Can you work these out from the drawing? Everything is in mm from the part's minimum corner. Round coordinates to 2 decimals unless told otherwise and drop trailing zeros. Loops run counter-clockwise (first coordinate to the right, second up) from the corner with the lowest first, then second, coordinate; pieces in that order, holes last. Notation, with made-up numbers: (57.25, -3.75) - (100.25, -3.75) arc R10 cw to (100.25, 3.25) - close; hole circle Ø6 at (37.5, 52.25). An arc over 180 degrees is marked (long way). Put each result on its own line as item: value. Start each with the question number.
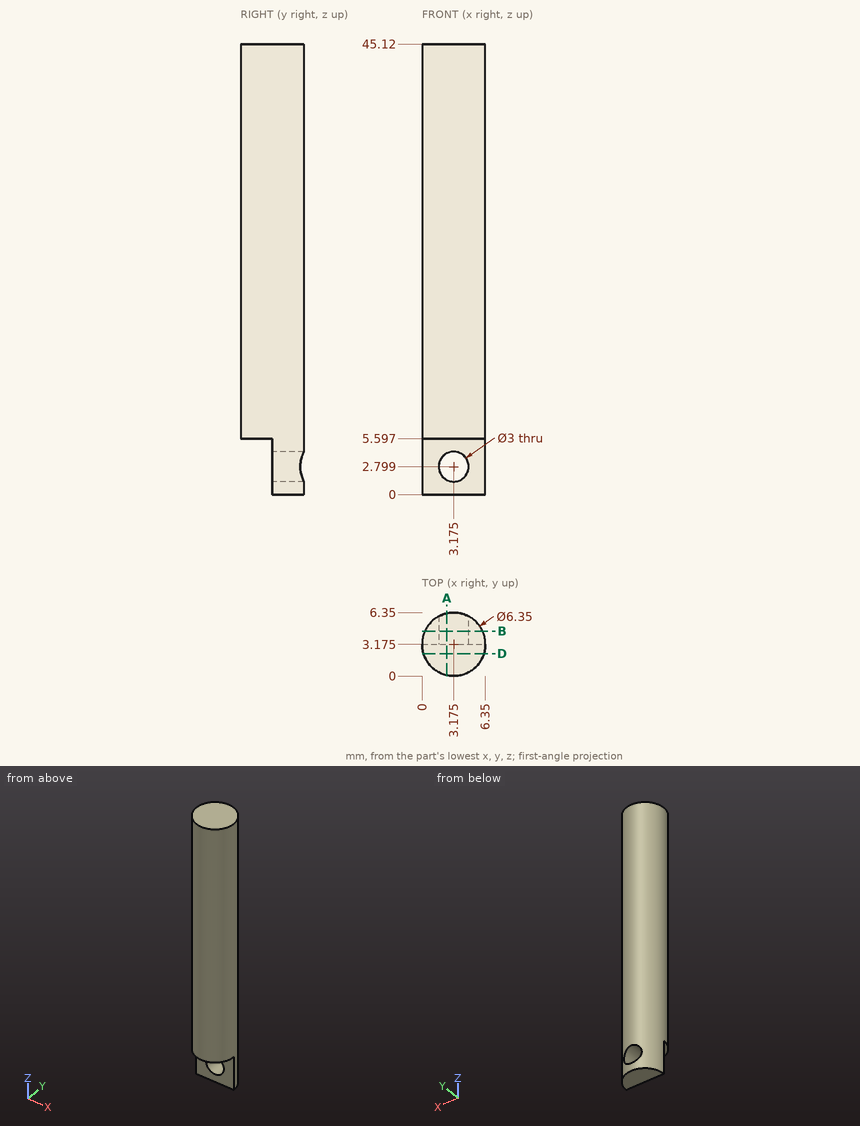
Item 1: Suppose I cut it at A-A, the plane x = 2.5. List the corners of the cut face in (y, z) for me (1 decimal), then the cut area to 3 significant figures.
Item 2: I need wall thicknesses on line 1 (Z direction, x = 1, y = 1.75); line 2 (Z direction, x = 3.75, y = 3.25) (1 decimal); line 3 (Z direction, x = 4.5, y = 3.5) (1 decimal). Which ranges of each line are inside material? Lowest first, please. Write a range as from..to.
Item 3: Suppose I cut it at B-B, the plane y = 4.5. List the corners of the cut face in (x, z) for me (1 decimal), then the cut area to 3 significant figures.
Item 4: Suppose I cut it at D-D, the plane y = 2.25. List the corners of the cut face in (x, z) for me, then the cut area to 3 significant figures.
Item 5: Will these pins go through, and if not, where does the flat tip stop? P1, Ø3.5, axis at x = 3.18, z = 2.8, coming from the -Y side (3 decimals); P2, Ø1, axis at x = 2.5, y = 1, coming from the -Z side; P3, Ø3, axis at x = 5.5, z = 18.5, coming from the -Y side.
Numbers:
1. outline: (0.1, 5.6) - (3.2, 5.6) - (3.2, 4.1) - (6.3, 4.1) - (6.3, 45.1) - (0.1, 45.1) - close; (3.2, 0) - (6.3, 0) - (6.3, 1.5) - (3.2, 1.5) - close
1. area: 254 mm^2
2. line 1: 5.6..45.12
2. line 2: 0..1.4, 4.2..45.1
2. line 3: 0..2.1, 3.5..45.1
3. outline: (0.3, 0) - (6.1, 0) - (6.1, 45.1) - (0.3, 45.1) - close; hole circle Ø3 at (3.2, 2.8)
3. area: 253 mm^2
4. outline: (0.14, 5.6) - (6.21, 5.6) - (6.21, 45.12) - (0.14, 45.12) - close
4. area: 240 mm^2
5. P1: y = 3.175
5. P2: z = 5.6
5. P3: y = 0.11
